```python
from build123d import *

# Parameters (mm, degrees)
F1_DEPTH = 152.4


# Not quite as in the source:
# - ends of sketch curves that miss each other by under 0.0002 mm in the source are joined


with BuildPart() as f1:
    # F0 (on Front) → F1 (new body)
    with BuildSketch(Plane.XZ):
        with BuildLine():
            Line((0.247523, 3.176651), (-11.1182404, 3.176651))
            Line((-11.1182404, 3.176651), (-11.1182404, -3.1766256))
            Line((-11.1182404, -3.1766256), (11.1182404, -3.1766256))
            ThreePointArc((11.1182404, -3.1766256), (8.7779959458, -0.3307242374), (5.2517548, 0.7376922))
            ThreePointArc((5.2517548, 0.7376922), (2.4682848878, 1.3798901975), (0.247523, 3.176651))
        make_face()
    extrude(amount=F1_DEPTH)


solid = f1.part
```
Geometry: final body of the model. Coordinates: model frame, mm. Round coordinates to 2 decimals unless told otherwise and drop trailing zeros. Write each loop counter-clockwise with the first axis right and the second up, starting at its lowest first coordinate (ties: lowest second). Pieces come first, ordered by that corner, then holes.
Item 1: Pin query (flat end, axial travel): P1, Ø3, axis at y = -110, z = -1, coming from the +X side. Return the tip coordinate at first contact, or that it passes through.
Item 2: Material intervals for L1, parallel to X at y = -65, z = 2.75; L2, parallel to X at y = -13, z = -1; L3, parallel to Z at x = 2.75, y = -116.5, sorted ascending.
Item 3: Section query C-C (x = 9.5). Return loops of the section in (y, z).
Item 4: Section query B-B (z = -1.5). Return loops of the section in (x, y).
Item 5: Section query A-A (y = -79.5). Return loops of the section in (x, z).
Completed:
1. P1: stops at x = 10.79
2. L1: x = -11.12 to 0.61
2. L2: x = -11.12 to 9.62
2. L3: z = -3.18 to 1.25
3. outline: (-152.4, -3.18) - (0, -3.18) - (0, -0.89) - (-152.4, -0.89) - close
4. outline: (-11.12, -152.4) - (10.09, -152.4) - (10.09, 0) - (-11.12, 0) - close
5. outline: (-11.12, -3.18) - (11.12, -3.18) arc R6.35 ccw to (5.25, 0.74) arc R6.35 cw to (0.25, 3.18) - (-11.12, 3.18) - close
